Study the drawing (mm; zero at the part's minimum x, y, z) and answer. A direction names the side the tool comes from. Coordinates: 2 decimals unless noted, no trailing zeros. Write each loop counter-clockwise with the first axis right and the second up, starting at its lowest first coordinate (ties: lowest second). Pieces come first, ordered by that corner, then holes. Notation, with made-up numbers: (87.5, 27) - (130.5, 27) arc R16 cw to (130.5, 35) - close; hole circle Ø2 at (-38, 84.5). An arc over 180 degrees is marked (long way). One line per item, written item: value.
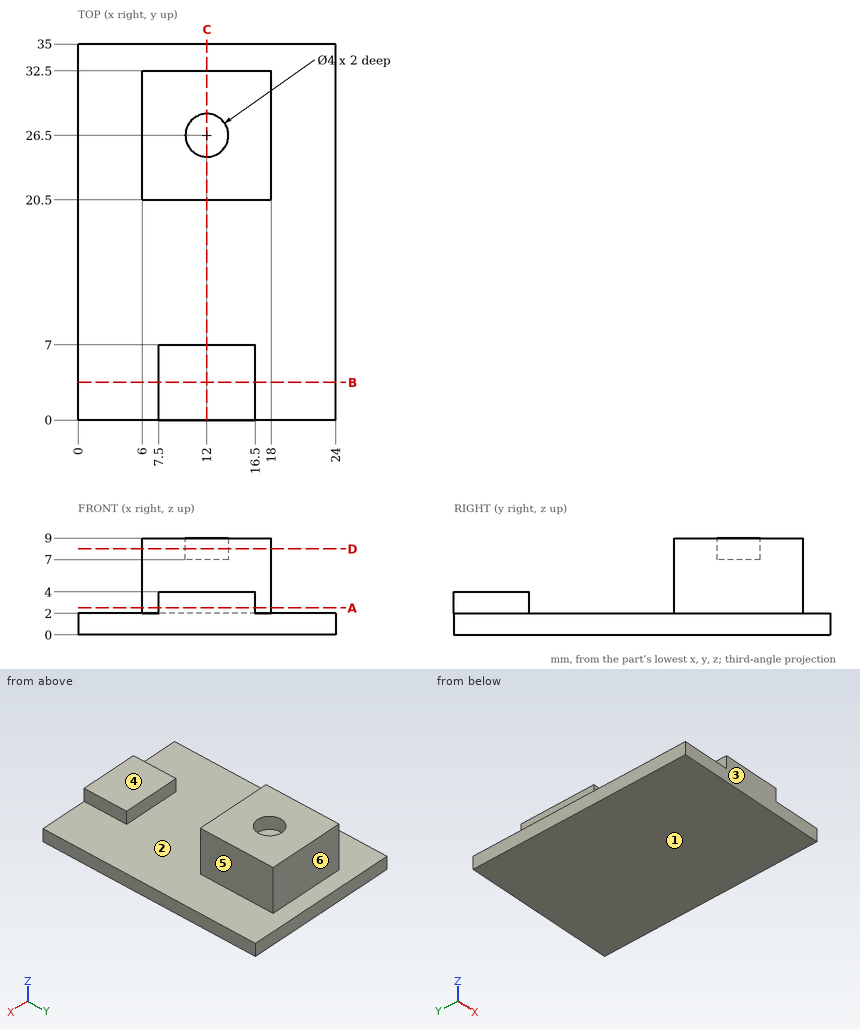
Item 1: Section C-C, the plane x = 12 is taken. Determine the outline of the cut face in (y, z).
Evaluation:
outline: (0, 0) - (35, 0) - (35, 2) - (32.5, 2) - (32.5, 9) - (28.5, 9) - (28.5, 7) - (24.5, 7) - (24.5, 9) - (20.5, 9) - (20.5, 2) - (7, 2) - (7, 4) - (0, 4) - close
Item 2: Given pin 1 (5.5 mm diameter, centred on x = 11.5, y = 5, fed in from +Z); pin 2 (3.5 mm diameter, centred on y = 28, z = 6, fed in from -X); pin 3 (5 mm diameter, centred on y = 25, z = 5, fed in from +X), each flat-ended and moving along its own axis, determine where each tip first touches the part or whether it passes through.
Evaluation:
pin 1: stops at z = 4
pin 2: stops at x = 6
pin 3: stops at x = 18
Item 3: Consider probe 1 along Y at (x, z) = (12, 8.35); probe 2 along Y at (x, z) = (14.75, 2.25); probe 3 along X at (y, z) = (30.5, 4). Determine where each line is inside the solid, lowest interval first.
Evaluation:
probe 1: y = 20.5 to 24.5, 28.5 to 32.5
probe 2: y = 0 to 7, 20.5 to 32.5
probe 3: x = 6 to 18
Item 4: Section A-A, the plane z = 2.5 is taken. Determine the outline of the cut face in (x, y).
Evaluation:
outline: (6, 20.5) - (18, 20.5) - (18, 32.5) - (6, 32.5) - close; (7.5, 0) - (16.5, 0) - (16.5, 7) - (7.5, 7) - close
Item 5: Section D-D, the plane z = 8 is taken. Determine the outline of the cut face in (x, y).
Evaluation:
outline: (6, 20.5) - (18, 20.5) - (18, 32.5) - (6, 32.5) - close; hole circle Ø4 at (12, 26.5)
Item 6: Which of the six approach directions +Z, -Z, +X, -X, +Y, -Y give full straight-line access (tool end or side, diameter ignored) to the marked faces 4, 5 and 6?
Evaluation:
face 4: +Z, +X, -X, -Y
face 5: +Z, +X, +Y, -Y
face 6: +Z, +X, -X, +Y
Item 7: Section B-B, the plane y = 3.5 is taken. Determine the outline of the cut face in (x, z), then the cut area to 3 significant figures.
Evaluation:
outline: (0, 0) - (24, 0) - (24, 2) - (16.5, 2) - (16.5, 4) - (7.5, 4) - (7.5, 2) - (0, 2) - close
area: 66.0 mm2
Item 8: Determine the mould class of the marked faces 1, 2 and 3 for opening direction Y: +Y half, -Y half, draft (parallel to the pull), parting line (faces both ways), or undercut.
Evaluation:
face 1: draft
face 2: undercut
face 3: -Y half
